from build123d import *

# Parameters (mm, degrees)
CROQUIS1_W              = 50
CROQUIS1_H              = 26
SALIENTE_EXTRUIR1_DEPTH = 1.5
CROQUIS2_W              = 7.5
CROQUIS2_H              = 15.5
SALIENTE_EXTRUIR2_DEPTH = 10
CHAFL_N1_SIZE           = 3
CHAFL_N1_SIZE2          = 1.732050808
CHAFL_N1_PART_2_SIZE    = 3
CHAFL_N1_PART_2_SIZE2   = 1.732050808
CHAFL_N1_PART_3_SIZE    = 3
CHAFL_N1_PART_3_SIZE2   = 1.732050808
CHAFL_N1_PART_4_SIZE    = 3
CHAFL_N1_PART_4_SIZE2   = 1.732050808
CROQUIS3_W              = 18.5
CROQUIS3_H              = 15.5
SALIENTE_EXTRUIR3_DEPTH = 15.5
CROQUIS4_W              = 30
CROQUIS4_H              = 15
SALIENTE_EXTRUIR4_DEPTH = 2
CROQUIS5_R              = 1.5
CORTAR_EXTRUIR1_DEPTH   = 2


with BuildPart() as part:
    # Croquis1 → Saliente-Extruir1 (new body)
    with BuildSketch(Plane(origin=(0, 0, 0), x_dir=(1, 0, 0), z_dir=(0, 1, 0))):
        Rectangle(CROQUIS1_W, CROQUIS1_H)
    extrude(amount=SALIENTE_EXTRUIR1_DEPTH)

    # Croquis2 → Saliente-Extruir2 (add)
    with BuildSketch(Plane(origin=(0, 1.5, 0), x_dir=(1, 0, 0), z_dir=(0, 1, 0))):
        with Locations((15.25, 0.25)):
            Rectangle(CROQUIS2_W, CROQUIS2_H)
        with Locations((-18.75, 0.25)):
            Rectangle(CROQUIS2_W, CROQUIS2_H)
    extrude(amount=SALIENTE_EXTRUIR2_DEPTH)

    # Chaflán1
    chafl_n1_edges = [part.edges().sort_by_distance(p)[0] for p in [
        (19, 11.5, -0.25),
    ]]
    chafl_n1_side = [part.faces().sort_by_distance(p)[0] for p in [
        (19, 6.5, -0.25),
    ]]
    chamfer(chafl_n1_edges, length=CHAFL_N1_SIZE, length2=CHAFL_N1_SIZE2, reference=chafl_n1_side[0])

    # Chaflán1 part 2
    chafl_n1_part_2_edges = [part.edges().sort_by_distance(p)[0] for p in [
        (11.5, 11.5, -0.25),
    ]]
    chafl_n1_part_2_side = [part.faces().sort_by_distance(p)[0] for p in [
        (11.5, 6.5, -0.25),
    ]]
    chamfer(chafl_n1_part_2_edges, length=CHAFL_N1_PART_2_SIZE, length2=CHAFL_N1_PART_2_SIZE2, reference=chafl_n1_part_2_side[0])

    # Chaflán1 part 3
    chafl_n1_part_3_edges = [part.edges().sort_by_distance(p)[0] for p in [
        (-15, 11.5, -0.25),
    ]]
    chafl_n1_part_3_side = [part.faces().sort_by_distance(p)[0] for p in [
        (-15, 6.5, -0.25),
    ]]
    chamfer(chafl_n1_part_3_edges, length=CHAFL_N1_PART_3_SIZE, length2=CHAFL_N1_PART_3_SIZE2, reference=chafl_n1_part_3_side[0])

    # Chaflán1 part 4
    chafl_n1_part_4_edges = [part.edges().sort_by_distance(p)[0] for p in [
        (-22.5, 11.5, -0.25),
    ]]
    chafl_n1_part_4_side = [part.faces().sort_by_distance(p)[0] for p in [
        (-22.5, 6.5, -0.25),
    ]]
    chamfer(chafl_n1_part_4_edges, length=CHAFL_N1_PART_4_SIZE, length2=CHAFL_N1_PART_4_SIZE2, reference=chafl_n1_part_4_side[0])

    # Croquis3 → Saliente-Extruir3 (add)
    with BuildSketch(Plane(origin=(0, 1.5, 0), x_dir=(1, 0, 0), z_dir=(0, 1, 0))):
        with Locations((2.25, 0.25)):
            Rectangle(CROQUIS3_W, CROQUIS3_H)
    extrude(amount=SALIENTE_EXTRUIR3_DEPTH)

    # Croquis4 → Saliente-Extruir4 (add)
    with BuildSketch(Plane.XZ):
        Rectangle(CROQUIS4_W, CROQUIS4_H)
    extrude(amount=SALIENTE_EXTRUIR4_DEPTH)

    # Croquis5 → Cortar-Extruir1 (cut)
    with BuildSketch(Plane.XZ):
        with Locations((-22.5, 10.75)):
            Circle(CROQUIS5_R)
        with Locations((22.5, 10.75)):
            Circle(CROQUIS5_R)
        with Locations((22.5, -10.5)):
            Circle(CROQUIS5_R)
        with Locations((-22.5, -10.5)):
            Circle(CROQUIS5_R)
    extrude(amount=-CORTAR_EXTRUIR1_DEPTH, mode=Mode.SUBTRACT)


solid = part.part
Verification items for the finished model (mm, model axes). A direction names the side the tool comes from. Coordinates: 2 decimals unless noted, no trailing zeros. Write each loop counter-clockwise with the first axis right and the second up, starting at its lowest first coordinate (ties: lowest second). Pieces come first, ordered by that corner, then holes. Notation, with made-up numbers: (51.5, 85.5) -> (100.5, 85.5) arc R21 cw to (100.5, 90.5) -> close; hole circle Ø11 at (-16, 5.25). An arc over 180 degrees is marked (long way). One line per item, written item: value. Start each with the question number.
Q1. Go/stop test with flat-tipped pins: P1, Ø6, axis at x = -17.5, y = 6, coming from the -Z side; P2, Ø1, axis at x = -3, y = -1, coming from the -Z side; P3, Ø6, axis at x = -13.5, y = 8, coming from the +Z side; P4, Ø1.8, axis at x = 22.5, z = -10.5, coming from the -Y side. Record where each tip stops, or that it passes through.
Q2. Access from +Z, -Z, +X, -X, +Y, -Y to the whole of each face (thin tool, end or side, straight path). Record for faces 1 (the flat face through (-15, -1, 0)), 2 (the flat face through (-22.5, 5, 0)), 3 (the flat face through (-19, 6, -8)), 4 (the flat face through (6, 9, 7.5)), 5 (the flat face through (15, -1, 0)).
Q3. Cross-section at B-B on x = 22.5. Enter the section's corners in (y, z).
Q4. Mould release check, pull along X, two halves, no side actions. Record for faces 6 (the flat face through (-7, 9, 0)), 7 (the flat face through (0, 1, 13)), 8 (the flat face through (25, 1, 0)), 9 (the flat face through (-25, 1, 0)): pulls with the +X half, pulls with the -X half, needs draft (parallel to the pull), parting line crosses it, or undercut.
Q5. Cross-section at C-C on y = 3.75. Enter the section's corners in (x, z).
Q6. Thickness scan on L1, parallel to Z at x = -22.5, y = 0.7; L2, parallel to X at y = 5, z = -1.75; L3, parallel to Z at x = 13.5, y = 2.5. Record the ranges inside material, lowest first. Write a range as from..to.
Q7. Cross-section at D-D on z = -5. Enter the section's corners in (x, y).
Q8. Cross-section at A-A on z = -10.5. Enter the section's corners in (x, y).
Checked values:
1. P1: stops at z = -8
1. P2: stops at z = -7.5
1. P3: stops at z = 7.5
1. P4: passes through
2. face 1: +Z, -Z, -X, -Y
2. face 2: +Z, -Z, -X, +Y
2. face 3: -Z, +X, -X, +Y
2. face 4: +Z, +X, -X, +Y
2. face 5: +Z, -Z, +X, -Y
3. outline: (0, -13) -> (1.5, -13) -> (1.5, -12) -> (0, -12) -> close; (0, -9) -> (1.5, -9) -> (1.5, 9.25) -> (0, 9.25) -> close; (0, 12.25) -> (1.5, 12.25) -> (1.5, 13) -> (0, 13) -> close
4. face 6: undercut
4. face 7: needs draft
4. face 8: pulls with the +X half
4. face 9: pulls with the -X half
5. outline: (-22.5, -8) -> (-15, -8) -> (-15, 7.5) -> (-22.5, 7.5) -> close; (-7, -8) -> (19, -8) -> (19, 7.5) -> (-7, 7.5) -> close
6. L1: z = -13..-12, -9..9.25, 12.25..13
6. L2: x = -22.5..-15, -7..19
6. L3: z = -8..7.5
7. outline: (-25, 0) -> (-15, 0) -> (-15, -2) -> (15, -2) -> (15, 0) -> (25, 0) -> (25, 1.5) -> (19, 1.5) -> (19, 8.5) -> (17.27, 11.5) -> (13.23, 11.5) -> (11.5, 8.5) -> (11.5, 17) -> (-7, 17) -> (-7, 1.5) -> (-15, 1.5) -> (-15, 8.5) -> (-16.73, 11.5) -> (-20.77, 11.5) -> (-22.5, 8.5) -> (-22.5, 1.5) -> (-25, 1.5) -> close
8. outline: (-25, 0) -> (-24, 0) -> (-24, 1.5) -> (-25, 1.5) -> close; (-21, 0) -> (21, 0) -> (21, 1.5) -> (-21, 1.5) -> close; (24, 0) -> (25, 0) -> (25, 1.5) -> (24, 1.5) -> close
